```python
from build123d import *

# Parameters (mm, degrees)
CROQUIS1_R              = 7.5
CROQUIS1_R_2            = 2
SALIENTE_EXTRUIR1_DEPTH = 4
CROQUIS2_R              = 2.193779366
SALIENTE_EXTRUIR2_DEPTH = 5
CROQUIS3_R              = 7.5
CROQUIS3_R_2            = 2
SALIENTE_EXTRUIR3_DEPTH = 4
CROQUIS4_R              = 2.193779366
CORTAR_EXTRUIR1_DEPTH   = 14
SALIENTE_EXTRUIR4_DEPTH = 13


with BuildPart() as part:
    # Croquis1 → Saliente-Extruir1 (new body)
    with BuildSketch(Plane.XY):
        Circle(CROQUIS1_R)
        Circle(CROQUIS1_R_2, mode=Mode.SUBTRACT)
    extrude(amount=SALIENTE_EXTRUIR1_DEPTH)



with BuildPart() as body_2:
    # Croquis2 → Saliente-Extruir2 (new body)
    with BuildSketch(Plane(origin=(0, 0, 0), x_dir=(-1, 0, 0), z_dir=(0, 0, -1))):
        Circle(CROQUIS2_R)
    extrude(amount=SALIENTE_EXTRUIR2_DEPTH)

    # Croquis4 → Cortar-Extruir1 (cut)
    with BuildSketch(Plane(origin=(0, 0, -5), x_dir=(-1, 0, 0), z_dir=(0, 0, -1))):
        Circle(CROQUIS4_R)
    extrude(amount=-CORTAR_EXTRUIR1_DEPTH, mode=Mode.SUBTRACT)


with BuildPart() as body_3:
    # Croquis3 → Saliente-Extruir3 (new body)
    with BuildSketch(Plane(origin=(0, 0, -5), x_dir=(-1, 0, 0), z_dir=(0, 0, -1))):
        Circle(CROQUIS3_R)
        Circle(CROQUIS3_R_2, mode=Mode.SUBTRACT)
    extrude(amount=SALIENTE_EXTRUIR3_DEPTH)


with BuildPart() as part_1:
    add(part.part)

    add(body_3.part)  # Saliente-Extruir4 merges body 3
    # Croquis5 → Saliente-Extruir4 (add)
    with BuildSketch(Plane.XY.offset(4)):
        with BuildLine():
            Line((-10.009282788, -8.566914266), (0, -7.5))
            ThreePointArc((0, -7.5), (-5.895156044, -4.636500319), (-7.288771435, 1.76743061))
            ThreePointArc((-7.288771435, 1.76743061), (-27.875344012, -0.49038836), (-46.981845806, 7.5))
            Line((-46.981845806, 7.5), (-46.981845806, 4.90393409))
            ThreePointArc((-46.981845806, 4.90393409), (-30.939741801, -8.539865418), (-10.009282788, -8.566914266))
        make_face()
    extrude(amount=-SALIENTE_EXTRUIR4_DEPTH)


solid = part_1.part
```
Build history of the part. All positions in model axes, mm. A direction names the side the tool comes from. Round coordinates to 2 decimals unless told otherwise and drop trailing zeros. Write each loop counter-clockwise with the first axis right and the second up, starting at its lowest first coordinate (ties: lowest second). Pieces come first, ordered by that corner, then holes. Notation, with made-up numbers: (-3.75, 78) - (47.25, 78) arc R9 cw to (47.25, 94) - close; hole circle Ø2 at (-1.75, -21.75). An arc over 180 degrees is marked (long way). Answer as CSV lines item,"result".
Q1. Tool access for faces 1 (the cylindrical face through (-5.836, -4.711, -2.465)), 2 (the flat face through (-5.07, -8.04, -2.41)): list every direction of +Z, -Z, +X, -X, +Y, -Y with a clear straight run to the whole face (end or side of a thin tool).
Report:
face 1,"+X"
face 2,"+Z, -Z, +X, -Y"
Q2. Pull direction Y, two halves, no side cores. Call faces 3 (the cylindrical face through (6.037, 4.45, 1.972)), 4 (the cylindrical face through (0, -2, 2)), 5 (the cylindrical face through (-31.22, -8.436, -2.409)): +Y half, -Y half, draft (parallel to the pull), parting line (faces both ways), or undercut.
Report:
face 3,"parting line"
face 4,"undercut"
face 5,"-Y half"
Q3. Cut at A-A (y = 0). Write the cut outline in (x, z), and give its area (3 significant figures).
Report:
outline,"(-43.45, -9) - (-30.62, -9) - (-30.62, 4) - (-43.45, 4) - close; (-13.29, -9) - (-2, -9) - (-2, -5) - (-7.5, -5) - (-7.5, 0) - (-2, 0) - (-2, 4) - (-13.29, 4) - close; (2, -9) - (7.5, -9) - (7.5, -5) - (2, -5) - close; (2, 0) - (7.5, 0) - (7.5, 4) - (2, 4) - close"
area,"330 mm^2"
Q4. Cut at C-C (z = -4.5). Write the cut outline in (x, y).
Report:
outline,"(-46.98, 4.9) arc R30.68 ccw to (-10.01, -8.57) - (0, -7.5) arc R7.5 cw to (-7.29, 1.77) arc R41.42 cw to (-46.98, 7.5) - close"
Q5. Cut at B-B (z = 0.5). Write the cut outline in (x, y), and give its area (3 significant figures).
Report:
outline,"(-46.98, 4.9) arc R30.68 ccw to (-10.01, -8.57) - (0, -7.5) arc R7.5 ccw (long way) to (-7.29, 1.77) arc R41.42 cw to (-46.98, 7.5) - close; hole circle Ø4 at (0, 0)"
area,"504 mm^2"
Q6. Drop flat-ended pins along their axis: pin 1 (1.5 mm diameter, centred on x = -15, z = -1, fed in from -Y); pin 2 (3 mm diameter, centred on y = -7.5, z = -6, fed in from -X); pin 3 (6 mm diameter, centred on x = -28.5, z = -4, fed in from +Y). Give the stop position or say it passes through.
Report:
pin 1,"stops at y = -10.03"
pin 2,"stops at x = -36.26"
pin 3,"stops at y = 0.2"
Q7. Drill centre lines: probe 1 along Y at (x, z) = (0, 1.3); probe 2 along Z at (x, y) = (-3, -0.5); probe 3 along Y at (x, z) = (-39.5, -3). Where is each one in solid material? Low to high. Write a range as [from, to].
Report:
probe 1,"y = [-7.5, -2], [2, 7.5]"
probe 2,"z = [-9, -5], [0, 4]"
probe 3,"y = [-3.75, 2.98]"
Q8. Cut at D-D (y = 6). Write the cut outline in (x, z).
Report:
outline,"(-46.98, -9) - (-44.87, -9) - (-44.87, 4) - (-46.98, 4) - close; (-4.5, -9) - (4.5, -9) - (4.5, -5) - (-4.5, -5) - close; (-4.5, 0) - (4.5, 0) - (4.5, 4) - (-4.5, 4) - close"
